Here's how the part is built. I have some questions about the finished solid (model axes, mm). A direction names the side the tool comes from. Coordinates: 2 decimals unless noted, no trailing zeros. Write each loop counter-clockwise with the first axis right and the second up, starting at its lowest first coordinate (ties: lowest second). Pieces come first, ordered by that corner, then holes. Notation, with made-up numbers: (-19, 88) -> (20, 88) arc R20 ccw to (20, 101) -> close; hole circle Ø8 at (29, -33.75). An arc over 180 degrees is marked (long way). Put each result on its own line as item: value.
```python
from build123d import *

# Parameters (mm, degrees)
SKETCH_1_W          = 45.073019954
SKETCH_1_H          = 60
SKETCH_1_R          = 1.525
EXTRUDE_1_DEPTH     = 3
SKETCH_2_W          = 10
SKETCH_2_H          = 60
EXTRUDE_2_DEPTH     = 10
HOLE_WIZARD_1_D     = 8.3
EXTRUDE_3_DEPTH     = 60
CUT_EXTRUDE_1_DEPTH = 0.7
HOLE_WIZARD_2_D     = 3
HOLE_WIZARD_2_DEPTH = 5


with BuildPart() as part:
    # 草图1 → 凸台-拉伸1 (new body)
    with BuildSketch(Plane.XY):
        with Locations((37.463490023, 30)):
            Rectangle(SKETCH_1_W, SKETCH_1_H)
        with Locations((20.831064203, 4.5)):
            Circle(SKETCH_1_R, mode=Mode.SUBTRACT)
        with Locations((50.351484989, 4.5)):
            Circle(SKETCH_1_R, mode=Mode.SUBTRACT)
        with Locations((20.926980046, 55.5)):
            Circle(SKETCH_1_R, mode=Mode.SUBTRACT)
        with Locations((50.351484989, 55.5)):
            Circle(SKETCH_1_R, mode=Mode.SUBTRACT)
    extrude(amount=EXTRUDE_1_DEPTH)

    # 草图2 → 凸台-拉伸2 (add)
    with BuildSketch(Plane.XY.offset(3)):
        with Locations((35.639232517, 30)):
            Rectangle(SKETCH_2_W, SKETCH_2_H)
    extrude(amount=EXTRUDE_2_DEPTH)

    # 孔1 (through all)
    with Locations(Plane(origin=(0, 0, 0), x_dir=(-1, 0, 0), z_dir=(0, -1, 0))):
        with Locations((-35.639232517, -5)):
            Hole(HOLE_WIZARD_1_D / 2)

    # 草图5 → 凸台-拉伸3 (add)
    with BuildSketch(Plane.XZ):
        Polygon((30.639232517, 13), (25.639232517, 3), (30.639232517, 3), align=None)
        Polygon((40.639232517, 13), (45.639232517, 3), (40.639232517, 3), align=None)
    extrude(amount=-EXTRUDE_3_DEPTH)

    # 草图7 → 切除-拉伸1 (cut, symmetric)
    with BuildSketch(Plane.XY.offset(11)):
        Polygon((37.313548298, 12.1), (38.987864079, 15), (37.313548298, 17.9), (33.964916737, 17.9), (32.290600956, 15), (33.964916737, 12.1), align=None)
        Polygon((38.987864079, 45), (37.313548298, 47.9), (33.964916737, 47.9), (32.290600956, 45), (33.964916737, 42.1), (37.313548298, 42.1), align=None)
    extrude(amount=CUT_EXTRUDE_1_DEPTH, both=True, mode=Mode.SUBTRACT)

    # 孔2
    with Locations(Plane.XY.offset(13)):
        with Locations((35.639232517, 45), (35.639232517, 15)):
            Hole(HOLE_WIZARD_2_D / 2, depth=HOLE_WIZARD_2_DEPTH)


solid = part.part
```
Item 1: Please list where these lines run through material, in increasing order: line 1 along Y through (x, z) = (36.5, 11.75); line 2 along Y through (x, z) = (35, 9.5); line 3 along Z through (x, y) = (46, 39). Write a range as from..to.
Output:
line 1: y = 0..13.77, 16.23..43.77, 46.23..60
line 2: y = 0..13.64, 16.36..43.64, 46.36..60
line 3: z = 0..3
Item 2: Imagine slicing it at B-B on x = 38. Write out the boundary of the cut face in (y, z), then the cut area to 3 significant figures.
Output:
outline: (0, 0) -> (60, 0) -> (60, 1.59) -> (0, 1.59) -> close; (0, 8.41) -> (60, 8.41) -> (60, 13) -> (0, 13) -> close; hole (13.29, 10.3) -> (16.71, 10.3) -> (16.71, 11.7) -> (13.29, 11.7) -> close; hole (43.29, 10.3) -> (46.71, 10.3) -> (46.71, 11.7) -> (43.29, 11.7) -> close
area: 361 mm²
Item 3: For P1, Ø1.8, axis at x = 20.93, y = 55.5, coming from the -Z side; P2, Ø2.5, axis at x = 35.64, y = 45, coming from the +Z side; P3, Ø8, axis at x = 46, y = 36.5, coming from the +Z side; P4, Ø3, axis at x = 22.5, y = 38.5, coming from the +Z side, each with a flat end and sliding along its axis, tell me the tip position at first contact or that it passes through.
Output:
P1: passes through
P2: stops at z = 1.04
P3: stops at z = 10.28
P4: stops at z = 3
Item 4: Imagine slicing it at D-D on z = 5. Write out the boundary of the cut face in (x, y).
Output:
outline: (26.64, 0) -> (31.49, 0) -> (31.49, 60) -> (26.64, 60) -> close; (39.79, 0) -> (44.64, 0) -> (44.64, 60) -> (39.79, 60) -> close
Item 5: If we mould it in two halves opening along Z, with no side actions, what happens to faces 1 (the cylindrical face through (36.83, 14.09, 12.34)), 2 (the flat face through (33.1, 13.6, 11)), 3 (the flat face through (20, 30, 3))? For each: released by +Z, released by -Z, zero draft, split by the parting line, or undercut.
Output:
face 1: zero draft
face 2: undercut
face 3: released by +Z
Item 6: Imagine slicing it at A-A on y = 4.5. Write out the boundary of the cut face in (x, z), then the cut area to 3 significant figures.
Output:
outline: (14.93, 0) -> (19.31, 0) -> (19.31, 3) -> (14.93, 3) -> close; (22.36, 0) -> (48.83, 0) -> (48.83, 3) -> (45.64, 3) -> (40.64, 13) -> (30.64, 13) -> (25.64, 3) -> (22.36, 3) -> close; (51.88, 0) -> (60, 0) -> (60, 3) -> (51.88, 3) -> close; hole circle Ø8.3 at (35.64, 5)
area: 213 mm²
Item 7: Imagine slicing it at C-C on y = 41. Write out the boundary of the cut face in (x, z), then the cut area to 3 significant figures.
Output:
outline: (14.93, 0) -> (60, 0) -> (60, 3) -> (45.64, 3) -> (40.64, 13) -> (30.64, 13) -> (25.64, 3) -> (14.93, 3) -> close; hole circle Ø8.3 at (35.64, 5)
area: 231 mm²
Item 8: Which directions (+Z, -Z, +X, -X, +Y, -Y) give clear straight access to the entire face, cutting with the end or side of a thin tool? Please do faces 4 (the cylindrical face through (35.964, 43.536, 12.341)), 5 (the flat face through (37.1, 0, 0.8)), 6 (the flat face through (33.14, 16.47, 10.99)).
Output:
face 4: +Z
face 5: +Z, -Z, +X, -X, -Y
face 6: none
